Geometry: final body of the model. Coordinates: model frame, mm. Face numbers are marked on the shaded views. Round coordinates to 2 decimals unless told otherwise and drop trailing zeros. Write each loop counter-clockwise with the first axis right and the second up, starting at its lowest first coordinate (ties: lowest second). Pieces come first, ordered by that corner, then holes. Notation, with made-up numbers: (9, 66) -> (14, 66) arc R23 cw to (14, 77) -> close; hole circle Ø10 at (-37.5, 60.5). An arc over 180 degrees is marked (long way). Use one line per item in the form item = value. Start each with the question number.
1. Line query: L1, parallel to Y at x = 0, z = 6; L2, parallel to X at y = -9.5, z = 20; L3, parallel to Y at x = -2, z = -7. Output: solid intervals per line, ascending.
2. Cut plane B-B, the plane x = 0. Return the cut outline in (y, z), plus the area to 3 significant figures.
3. Draft query along X for the marked faces 1 and 2. Return one class per face: pulls with the +X half, pulls with the -X half, needs draft (parallel to the pull), parting line crosses it, or undercut.
4. Cut plane D-D, the plane x = 19. Return the cut outline in (y, z), plus the area to 4 significant figures.
5. Cut plane A-A, the plane z = 22.5. Return the cut outline in (x, y), plus the area to 3 significant figures.
6. Pin query (flat end, axial travel): pin 1 Ø12 at (x, z) = (-2.5, 23.5) entering from -Y; pin 2 Ø6 at (x, y) = (-4, 13.5) entering from +Z; pin 3 Ø10 at (y, z) = (23.5, 3.5) entering from +X; pin 4 Ø2.5 at (y, z) = (-22, 1) entering from -X. Return the tip coordinate at first contact, or that it passes through.
7. Cut plane C-C, the plane y = -23. Return the cut outline in (x, z).
```python
from build123d import *

# Parameters (mm, degrees)
F0_R     = 16
F1_DEPTH = 32.5
F0_R_2   = 28
F2_DEPTH = 32.5


with BuildPart() as f1:
    # F0 (on Top) → F1 (new body, symmetric)
    with BuildSketch(Plane.XY):
        with BuildLine():
            ThreePointArc((15.7417332781, -7.6451182726), (17.0547696022, -3.9223505474), (17.5, 0))
            ThreePointArc((17.5, 0), (17.0547696022, 3.9223505474), (15.7417332781, 7.6451182726))
            ThreePointArc((15.7417332781, 7.6451182726), (15.1554445662, 8.75), (14.4917332781, 9.8101817821))
            ThreePointArc((14.4917332781, 9.8101817821), (8.75, 15.1554445662), (1.25, 17.4553000547))
            ThreePointArc((1.25, 17.4553000547), (0, 17.5), (-1.25, 17.4553000547))
            ThreePointArc((-1.25, 17.4553000547), (-8.75, 15.1554445662), (-14.4917332781, 9.8101817821))
            ThreePointArc((-14.4917332781, 9.8101817821), (-15.1554445662, 8.75), (-15.7417332781, 7.6451182726))
            ThreePointArc((-15.7417332781, 7.6451182726), (-17.5, 0), (-15.7417332781, -7.6451182726))
            ThreePointArc((-15.7417332781, -7.6451182726), (-15.1554445662, -8.75), (-14.4917332781, -9.8101817821))
            ThreePointArc((-14.4917332781, -9.8101817821), (-8.75, -15.1554445662), (-1.25, -17.4553000547))
            ThreePointArc((-1.25, -17.4553000547), (0, -17.5), (1.25, -17.4553000547))
            ThreePointArc((1.25, -17.4553000547), (8.75, -15.1554445662), (14.4917332781, -9.8101817821))
            ThreePointArc((14.4917332781, -9.8101817821), (15.1554445662, -8.75), (15.7417332781, -7.6451182726))
        make_face()
        Circle(F0_R, mode=Mode.SUBTRACT)
    extrude(amount=F1_DEPTH, both=True)



with BuildPart() as f1b:
    # F0 (on Top) → F1, piece 2 (new body, symmetric)
    with BuildSketch(Plane.XY):
        Circle(F0_R_2)
        with BuildLine():
            ThreePointArc((22.2991275734, 14.3177829802), (22.9496732003, 13.25), (23.5491275734, 12.1527194707))
            ThreePointArc((23.5491275734, 12.1527194707), (25.751717231, 6.2529240882), (26.5, 0))
            ThreePointArc((26.5, 0), (25.751717231, -6.2529240882), (23.5491275734, -12.1527194707))
            ThreePointArc((23.5491275734, -12.1527194707), (22.9496732003, -13.25), (22.2991275734, -14.3177829802))
            ThreePointArc((22.2991275734, -14.3177829802), (13.25, -22.9496732003), (1.25, -26.4705024508))
            ThreePointArc((1.25, -26.4705024508), (0, -26.5), (-1.25, -26.4705024508))
            ThreePointArc((-1.25, -26.4705024508), (-13.25, -22.9496732003), (-22.2991275734, -14.3177829802))
            ThreePointArc((-22.2991275734, -14.3177829802), (-22.9496732003, -13.25), (-23.5491275734, -12.1527194707))
            ThreePointArc((-23.5491275734, -12.1527194707), (-26.5, 0), (-23.5491275734, 12.1527194707))
            ThreePointArc((-23.5491275734, 12.1527194707), (-22.9496732003, 13.25), (-22.2991275734, 14.3177829802))
            ThreePointArc((-22.2991275734, 14.3177829802), (-13.25, 22.9496732003), (-1.25, 26.4705024508))
            ThreePointArc((-1.25, 26.4705024508), (0, 26.5), (1.25, 26.4705024508))
            ThreePointArc((1.25, 26.4705024508), (13.25, 22.9496732003), (22.2991275734, 14.3177829802))
        make_face(mode=Mode.SUBTRACT)
    extrude(amount=F1_DEPTH, both=True)


with BuildPart() as f1_1:
    add(f1.part)

    add(f1b.part)  # F2 merges F1b
    # F0 (on Top) → F2 (join, symmetric)
    with BuildSketch(Plane.XY):
        with BuildLine():
            ThreePointArc((-15.7417332781, 7.6451182726), (-15.1554445662, 8.75), (-14.4917332781, 9.8101817821))
            Line((-14.4917332781, 9.8101817821), (-22.2991275734, 14.3177829802))
            ThreePointArc((-22.2991275734, 14.3177829802), (-22.9496732003, 13.25), (-23.5491275734, 12.1527194707))
            Line((-23.5491275734, 12.1527194707), (-15.7417332781, 7.6451182726))
        make_face()
        with BuildLine():
            ThreePointArc((-1.25, 17.4553000547), (0, 17.5), (1.25, 17.4553000547))
            Line((1.25, 17.4553000547), (1.25, 26.4705024508))
            ThreePointArc((1.25, 26.4705024508), (0, 26.5), (-1.25, 26.4705024508))
            Line((-1.25, 26.4705024508), (-1.25, 17.4553000547))
        make_face()
        with BuildLine():
            ThreePointArc((14.4917332781, 9.8101817821), (15.1554445662, 8.75), (15.7417332781, 7.6451182726))
            Line((15.7417332781, 7.6451182726), (23.5491275734, 12.1527194707))
            ThreePointArc((23.5491275734, 12.1527194707), (22.9496732003, 13.25), (22.2991275734, 14.3177829802))
            Line((22.2991275734, 14.3177829802), (14.4917332781, 9.8101817821))
        make_face()
        with BuildLine():
            Line((23.5491275734, -12.1527194707), (15.7417332781, -7.6451182726))
            ThreePointArc((15.7417332781, -7.6451182726), (15.1554445662, -8.75), (14.4917332781, -9.8101817821))
            Line((14.4917332781, -9.8101817821), (22.2991275734, -14.3177829802))
            ThreePointArc((22.2991275734, -14.3177829802), (22.9496732003, -13.25), (23.5491275734, -12.1527194707))
        make_face()
        with BuildLine():
            Line((1.25, -26.4705024508), (1.25, -17.4553000547))
            ThreePointArc((1.25, -17.4553000547), (0, -17.5), (-1.25, -17.4553000547))
            Line((-1.25, -17.4553000547), (-1.25, -26.4705024508))
            ThreePointArc((-1.25, -26.4705024508), (0, -26.5), (1.25, -26.4705024508))
        make_face()
        with BuildLine():
            Line((-22.2991275734, -14.3177829802), (-14.4917332781, -9.8101817821))
            ThreePointArc((-14.4917332781, -9.8101817821), (-15.1554445662, -8.75), (-15.7417332781, -7.6451182726))
            Line((-15.7417332781, -7.6451182726), (-23.5491275734, -12.1527194707))
            ThreePointArc((-23.5491275734, -12.1527194707), (-22.9496732003, -13.25), (-22.2991275734, -14.3177829802))
        make_face()
    extrude(amount=F2_DEPTH, both=True)


solid = f1_1.part
```
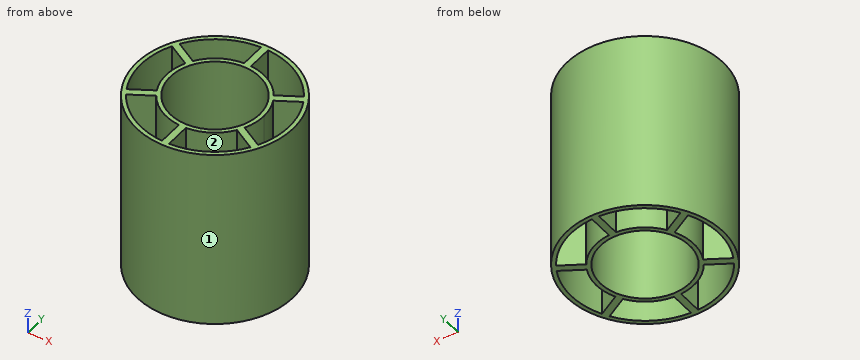
Outcome:
q1.L1 = -28 to -16, 16 to 28
q1.L2 = -26.34 to -24.74, -18.95 to -12.87, 12.87 to 18.95, 24.74 to 26.34
q1.L3 = -27.93 to -26.42, -17.39 to -15.87, 15.87 to 17.39, 26.42 to 27.93
q2.outline = (-28, -32.5) -> (-16, -32.5) -> (-16, 32.5) -> (-28, 32.5) -> close; (16, -32.5) -> (28, -32.5) -> (28, 32.5) -> (16, 32.5) -> close
q2.area = 1,560 mm^2
q3.face_1 = parting line crosses it
q3.face_2 = undercut
q4.outline = (-20.57, -32.5) -> (-18.47, -32.5) -> (-18.47, 32.5) -> (-20.57, 32.5) -> close; (-12.41, -32.5) -> (-9.53, -32.5) -> (-9.53, 32.5) -> (-12.41, 32.5) -> close; (9.53, -32.5) -> (12.41, -32.5) -> (12.41, 32.5) -> (9.53, 32.5) -> close; (18.47, -32.5) -> (20.57, -32.5) -> (20.57, 32.5) -> (18.47, 32.5) -> close
q4.area = 647.5 mm^2
q5.outline = circle Ø56 at (0, 0); hole (-23.55, -12.15) -> (-15.74, -7.65) arc R17.5 cw to (-15.74, 7.65) -> (-23.55, 12.15) arc R26.5 ccw to start; hole (-22.3, -14.32) arc R26.5 ccw to (-1.25, -26.47) -> (-1.25, -17.46) arc R17.5 cw to (-14.49, -9.81) -> close; hole (-22.3, 14.32) -> (-14.49, 9.81) arc R17.5 cw to (-1.25, 17.46) -> (-1.25, 26.47) arc R26.5 ccw to start; hole circle Ø32 at (0, 0); hole (1.25, -26.47) arc R26.5 ccw to (22.3, -14.32) -> (14.49, -9.81) arc R17.5 cw to (1.25, -17.46) -> close; hole (1.25, 17.46) arc R17.5 cw to (14.49, 9.81) -> (22.3, 14.32) arc R26.5 ccw to (1.25, 26.47) -> close; hole (15.74, -7.65) -> (23.55, -12.15) arc R26.5 ccw to (23.55, 12.15) -> (15.74, 7.65) arc R17.5 cw to start
q5.area = 550 mm^2
q6.pin_1 = -28
q6.pin_2 = 32.5
q6.pin_3 = 21.02
q6.pin_4 = -18.8
q7.outline = (-15.97, -32.5) -> (-13.16, -32.5) -> (-13.16, 32.5) -> (-15.97, 32.5) -> close; (-1.25, -32.5) -> (1.25, -32.5) -> (1.25, 32.5) -> (-1.25, 32.5) -> close; (13.16, -32.5) -> (15.97, -32.5) -> (15.97, 32.5) -> (13.16, 32.5) -> close
